```python
from build123d import *

# Parameters (mm, degrees)
F0_R     = 7.9375
F1_DEPTH = 139.7
F4_DEPTH = 2.38125
F5_SIZE  = 1.524


with BuildPart() as f1:
    # F0 (on Right) → F1 (new body, symmetric)
    with BuildSketch(Plane.YZ):
        Circle(F0_R)
    extrude(amount=F1_DEPTH, both=True)

    # F3 (on offset) → F4 (cut)
    with BuildSketch(Plane.XY.offset(7.9375)):
        with BuildLine():
            ThreePointArc((-116.6876, -2.38125), (-115.0038019773, -1.6837980227), (-114.30635, 0))
            ThreePointArc((-114.30635, 0), (-115.0038019773, 1.6837980227), (-116.6876, 2.38125))
            ThreePointArc((-116.6876, 2.38125), (-119.06885, 0), (-116.6876, -2.38125))
        make_face()
        with BuildLine():
            ThreePointArc((-116.6876, -2.38125), (-119.06885, 0), (-116.6876, 2.38125))
            Line((-116.6876, 2.38125), (-139.7, 2.38125))
            Line((-139.7, 2.38125), (-139.7, -2.38125))
            Line((-139.7, -2.38125), (-116.6876, -2.38125))
        make_face()
        with BuildLine():
            ThreePointArc((116.6876, -2.38125), (118.3713980227, -1.6837980227), (119.06885, 0))
            ThreePointArc((119.06885, 0), (118.3713980227, 1.6837980227), (116.6876, 2.38125))
            Line((116.6876, 2.38125), (116.6876, -2.38125))
        make_face()
        with BuildLine():
            ThreePointArc((116.6876, 2.38125), (118.3713980227, 1.6837980227), (119.06885, 0))
            ThreePointArc((119.06885, 0), (118.3713980227, -1.6837980227), (116.6876, -2.38125))
            Line((116.6876, -2.38125), (139.7, -2.38125))
            Line((139.7, -2.38125), (139.7, 2.38125))
            Line((139.7, 2.38125), (116.6876, 2.38125))
        make_face()
        with BuildLine():
            Line((116.6876, -2.38125), (116.6876, 2.38125))
            ThreePointArc((116.6876, 2.38125), (114.30635, 0), (116.6876, -2.38125))
        make_face()
    extrude(amount=-F4_DEPTH, mode=Mode.SUBTRACT)

    # F5
    f5_edges = [f1.edges().sort_by_distance(p)[0] for p in [
        (-139.7, -4.695888, -6.399417),
        (139.7, -4.695888, -6.399417),
    ]]
    chamfer(f5_edges, length=F5_SIZE)


solid = f1.part
```
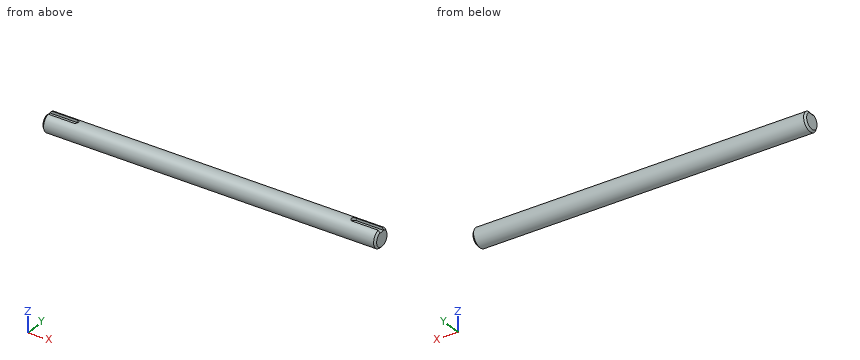
The model under review builds one solid part; all positions refer to its coordinate system, in mm. Give positions to 0.01 mm unless a question says otherwise; leave off trailing zeros. Write each loop counter-clockwise with the first axis right and the second up, starting at its lowest first coordinate (ties: lowest second). Pieces come first, ordered by that corner, then holes.
(1) For P1, Ø1, axis at x = 1.5, z = 3, coming from the -Y side; P2, Ø2, axis at x = -130.5, z = 6.5, coming from the +Y side; P3, Ø4, axis at x = 131.5, y = -0.5, coming from the +Z side; P4, Ø4, axis at x = 49, z = 0.5, coming from the +Y side, all flat-tipped, find the tip position at first contact; note any pin that passes through.
(2) Consider section A-A, the plane y = 0. Give the boundary of the cut face in (x, z).
(3) To check wall thickness, follow L1, parallel to X at y = 0.5, z = 5.75; L2, parallel to Y at x = -120, z = 6.5; L3, parallel to Z at x = -88.5, y = 0.25. State the ranges of each line that lie inside material, in increasing order.
(4) Consider section B-B, the plane x = -81. Give the boundary of the cut face in (y, z) (1 decimal).
Returned:
1. P1: stops at y = -7.53
1. P2: stops at y = 5.72
1. P3: stops at z = 7.57
1. P4: stops at y = 7.94
2. outline: (-139.7, -6.41) - (-138.18, -7.94) - (138.18, -7.94) - (139.7, -6.41) - (139.7, 5.56) - (114.31, 5.56) - (114.31, 7.94) - (-114.31, 7.94) - (-114.31, 5.56) - (-139.7, 5.56) - close
3. L1: x = -114.36 to 114.36
3. L2: y = -4.56 to -2.38, 2.38 to 4.56
3. L3: z = -7.93 to 7.93
4. outline: circle Ø15.9 at (0, 0)
